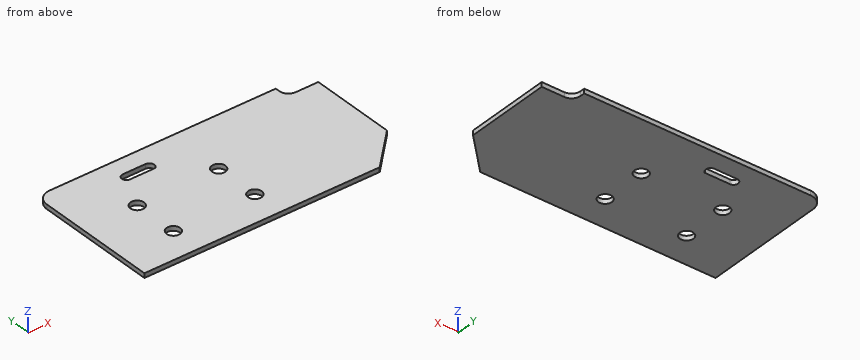
```python
from build123d import *

# Parameters (mm, degrees)
F1_DEPTH = 25.4
F2_D     = 76.2
F3_R     = 76.2
F4_SIZE  = 203.2
F5_R     = 50.8
F7_DEPTH = 25.401


with BuildPart() as f1:
    # F0 (on Top) → F1 (new body)
    with BuildSketch(Plane.XY):
        Polygon((0, 762), (0, 0), (1524, 0), (1524, 685.8), (1346.2, 685.8), (1346.2, 762), align=None)
    extrude(amount=F1_DEPTH)

    # F2 (through all)
    with Locations(Plane(origin=(0, 0, 0), x_dir=(1, 0, 0), z_dir=(0, 0, -1))):
        with Locations((304.8, -177.8), (304.8, -431.8), (762, -431.8), (762, -177.8)):
            Hole(F2_D / 2)

    # F3
    f3_edges = [f1.edges().sort_by_distance(p)[0] for p in [
        (0, 762, 12.7),
    ]]
    fillet(f3_edges, radius=F3_R)

    # F4
    f4_edges = [f1.edges().sort_by_distance(p)[0] for p in [
        (1524, 0, 12.7),
    ]]
    chamfer(f4_edges, length=F4_SIZE)

    # F5
    f5_edges = [f1.edges().sort_by_distance(p)[0] for p in [
        (1346.2, 685.8, 12.7),
    ]]
    fillet(f5_edges, radius=F5_R)

    # F6 (on Top) → F7 (cut, through all)
    with BuildSketch(Plane.XY):
        with BuildLine():
            Line((533.4, 660.4), (406.4, 660.4))
            ThreePointArc((406.4, 660.4), (381, 635), (406.4, 609.6))
            Line((406.4, 609.6), (547.8161634918, 609.6))
            ThreePointArc((547.8161634918, 609.6), (559.802962759, 640.4471760412), (533.4, 660.4))
        make_face()
    extrude(amount=F7_DEPTH, mode=Mode.SUBTRACT)


solid = f1.part
```
Geometry check sheet. Reference: the model listing, model coordinates, mm. Round coordinates to 2 decimals unless told otherwise and drop trailing zeros. Order: outer loops, then holes, each group sorted by start corner. A loop starts at its lowest first (then second) coordinate and runs counter-clockwise, first axis right, second up. Notation, with made-up numbers: (22, -19) - (28, -19) arc R5 ccw to (28, -15) - close; hole circle Ø5 at (86, -13). An arc over 180 degrees is marked (long way). Use a Markdown table: item, result. Add a question column.
(1) Material ranges on line 1 along Y through (x, z) = (762, 13); line 2 along X through (y, z) = (431.8, 8); line 3 along X through (y, z) = (450, 10.5), recorded low to high. Write a range as [from, to].
(2) Sectioned sample at B-B, the plane x = 444. Enter the section's corners in (y, z).
(3) Sectioned sample at D-D, the plane y = 635. Enter the section's corners in (x, z).
(4) Sectioned sample at A-A, the plane y = 431.8. Enter the section's corners in (x, z).
(5) Sectioned sample at C-C, the plane z = 20.5. Enter the section's corners in (x, y), and give its area (3 significant figures).
(6) Depth check by flat-ended pin: pin 1 (12 mm diameter, centred on y = 127.5, z = 6.5, fed in from +X); pin 2 (12 mm diameter, centred on x = 1332.5, y = 366, fed in from -Z); pin 3 (12.5 mm diameter, centred on y = 749.5, z = 8, fed in from +X). Enter the tip coordinate at first touch or a pass-through.
Answers below:
| question | item | result |
|---|---|---|
| 1 | line 1 | [0, 139.7], [215.9, 393.7], [469.9, 762] |
| 1 | line 2 | [0, 266.7], [342.9, 723.9], [800.1, 1524] |
| 1 | line 3 | [0, 271.33], [338.27, 728.53], [795.47, 1524] |
| 2 | outline | (0, 0) - (609.6, 0) - (609.6, 25.4) - (0, 25.4) - close; (660.4, 0) - (762, 0) - (762, 25.4) - (660.4, 25.4) - close |
| 3 | outline | (0, 0) - (381, 0) - (381, 25.4) - (0, 25.4) - close; (560.77, 0) - (1524, 0) - (1524, 25.4) - (560.77, 25.4) - close |
| 4 | outline | (0, 0) - (266.7, 0) - (266.7, 25.4) - (0, 25.4) - close; (342.9, 0) - (723.9, 0) - (723.9, 25.4) - (342.9, 25.4) - close; (800.1, 0) - (1524, 0) - (1524, 25.4) - (800.1, 25.4) - close |
| 5 | outline | (0, 0) - (1320.8, 0) - (1524, 203.2) - (1524, 685.8) - (1397, 685.8) arc R50.8 cw to (1346.2, 736.6) - (1346.2, 762) - (76.2, 762) arc R76.2 ccw to (0, 685.8) - close; hole circle Ø76.2 at (304.8, 177.8); hole circle Ø76.2 at (304.8, 431.8); hole (406.4, 609.6) - (547.82, 609.6) arc R27.45 ccw to (533.4, 660.4) - (406.4, 660.4) arc R25.4 ccw to start; hole circle Ø76.2 at (762, 177.8); hole circle Ø76.2 at (762, 431.8) |
| 5 | area | 1,100,000 mm² |
| 6 | pin 1 | x = 1454.3 |
| 6 | pin 2 | z = 0 |
| 6 | pin 3 | x = 1346.2 |
